Autodesk Inventor part; units mm, degrees
ref_plane "YZ Plane" through (0, 0, 0) normal (1, 0, 0) x (0, 1, 0)
ref_plane "XZ Plane" through (0, 0, 0) normal (0, 1, 0) x (-1, 0, 0)
ref_plane "XY Plane" through (0, 0, 0) normal (0, 0, 1) x (1, 0, 0)
sketch "Sketch1" plane through (0, 0, 0) normal (1, 0, 0) x (0, 1, 0)
  line L0 (-140, 0) -> (140, 0) construction
  line L1 (0, -2) -> (0, 12) construction
  line L2 (-100, 10) -> (100, 10)
  line L3 (100, 10) -> (100, 0)
  line L4 (100, 0) -> (-100, 0)
  line L5 (-100, 0) -> (-100, 10)
  point P0 (0, 0)
  dimension "d0" = 20
  dimension "d1" = 200
revolve "Revolution1" add sketch "Sketch1" angle 360 about axis through (0, -10, 0) along (0, 1, 0)
sketch "Sketch2" plane through (0, -100, 0) normal (0, -1, 0) x (1, 0, 0)
  circle A0 centre (0, 0) radius 10
hole "Hole1" at (0, -100, 0) direction (0, 1, 0) diameter 4.917 depth 20 tip angle 118
chamfer "Chamfer1" distance 0.5 angle 45 2 edges at (0, -100, -10) (0, 100, -10)
properties part number "DLT-01-236B" material "Aço SAE 1045"
The listing builds one solid part. Answer for the finished solid, in the listing's coordinates (mm). Coordinates: 2 decimals unless noted, no trailing zeros. Write each loop counter-clockwise with the first axis right and the second up, starting at its lowest first coordinate (ties: lowest second). Pieces come first, ordered by that corner, then holes.
Q1. The mould has two halves that part along Z. Classify faces 1 (the conical face through (0.13, -78.78, -0.41)), 2 (the flat face through (-2, -100, 2)), 3 (the cylindrical face through (-9.76, 1.39, -2.17)), 4 (the cylindrical face through (-0.738, -89.86, -2.345)): released by +Z, released by -Z, zero draft, split by the parting line, or undercut.
Returned:
face 1: undercut
face 2: zero draft
face 3: split by the parting line
face 4: undercut
Q2. Section A-A, the plane y = 75 is taken. Write down the section's boundary in (x, z), then the cut area to 3 significant figures.
Returned:
outline: circle Ø20 at (0, 0)
area: 314 mm2
Q3. Given P1, Ø5, axis at x = -7.5, y = 24.5, coming from the +Z side; P2, Ø1.5, axis at x = 6.5, y = 6.5, coming from the -Z side; P3, Ø10, axis at y = 2, z = -6.5, coming from the -X side, each flat-ended and moving along its own axis, determine where each tip first touches the part or whether it passes through.
Returned:
P1: stops at z = 8.66
P2: stops at z = -8.18
P3: stops at x = -9.89
Q4. Find the intervals of material crossed by line 1 along X through (y, z) = (-89.25, 0); line 2 along X through (y, z) = (0.5, -3); line 3 along Z through (x, y) = (-0.5, 51), in increasing order.
Returned:
line 1: x = -10 to -2.46, 2.46 to 10
line 2: x = -9.54 to 9.54
line 3: z = -9.99 to 9.99
